Work out the finished part from the listing and answer in its coordinate system (mm). A direction names the side the tool comes from. Round coordinates to 2 decimals unless told otherwise and drop trailing zeros. Order: outer loops, then holes, each group sorted by start corner. A loop starts at its lowest first (then second) coordinate and runs counter-clockwise, first axis right, second up. Notation, with made-up numbers: (-4.75, -14.5) - (36.25, -14.5) arc R32 cw to (36.25, 14.5) - close; hole circle Ø5 at (3, 74). An arc over 180 degrees is marked (long way). Put each result on its own line as item: value.
```python
from build123d import *

# Parameters (mm, degrees)
CROQUIS1_W              = 55
CROQUIS1_H              = 55
SALIENTE_EXTRUIR1_DEPTH = 180
CROQUIS2_R              = 6
CORTAR_EXTRUIR1_DEPTH   = 30
CROQUIS3_R              = 4
CORTAR_EXTRUIR2_DEPTH   = 25
CROQUIS4_R              = 2.5
CORTAR_EXTRUIR3_DEPTH   = 15
CORTAR_EXTRUIR4_START   = -15
CROQUIS5_R              = 2.5
CORTAR_EXTRUIR4_DEPTH   = 15
CROQUIS6_R              = 6
CORTAR_EXTRUIR5_DEPTH   = 12
CHAFL_N1_SIZE           = 2


with BuildPart() as part:
    # Croquis1 → Saliente-Extruir1 (new body)
    with BuildSketch(Plane.XY):
        Rectangle(CROQUIS1_W, CROQUIS1_H)
    extrude(amount=-SALIENTE_EXTRUIR1_DEPTH)

    # Croquis2 → Cortar-Extruir1 (cut)
    with BuildSketch(Plane.XY):
        Circle(CROQUIS2_R)
    extrude(amount=-CORTAR_EXTRUIR1_DEPTH, mode=Mode.SUBTRACT)

    # Croquis3 → Cortar-Extruir2 (cut)
    with BuildSketch(Plane(origin=(0, 0, -180), x_dir=(-1, 0, 0), z_dir=(0, 0, -1))):
        with Locations((18, 18)):
            Circle(CROQUIS3_R)
        with Locations((-18, 18)):
            Circle(CROQUIS3_R)
        with Locations((-18, -18)):
            Circle(CROQUIS3_R)
        with Locations((18, -18)):
            Circle(CROQUIS3_R)
    extrude(amount=-CORTAR_EXTRUIR2_DEPTH, mode=Mode.SUBTRACT)

    # Croquis4 → Cortar-Extruir3 (cut)
    with BuildSketch(Plane(origin=(27.5, 0, 0), x_dir=(0, 0, -1), z_dir=(1, 0, 0))):
        with Locations(Location((18, 21.5, 0), (0, 0, 90))):
            Circle(CROQUIS4_R)
        with Locations(Location((40, 21.5, 0), (0, 0, 90))):
            Circle(CROQUIS4_R)
        with Locations(Location((40, -21.5, 0), (0, 0, 90))):
            Circle(CROQUIS4_R)
        with Locations(Location((18, -21.5, 0), (0, 0, 90))):
            Circle(CROQUIS4_R)
    extrude(amount=-CORTAR_EXTRUIR3_DEPTH, mode=Mode.SUBTRACT)

    # Croquis5 → Cortar-Extruir4 (cut)
    with BuildSketch(Plane.ZY.offset(27.5).offset(CORTAR_EXTRUIR4_START)):
        with Locations(Location((-18, 21.5, 0), (0, 0, 90))):
            Circle(CROQUIS5_R)
        with Locations(Location((-40, 21.5, 0), (0, 0, 90))):
            Circle(CROQUIS5_R)
        with Locations(Location((-40, -21.5, 0), (0, 0, 90))):
            Circle(CROQUIS5_R)
        with Locations(Location((-18, -21.5, 0), (0, 0, 90))):
            Circle(CROQUIS5_R)
    extrude(amount=CORTAR_EXTRUIR4_DEPTH, mode=Mode.SUBTRACT)

    # Croquis6 → Cortar-Extruir5 (cut)
    with BuildSketch(Plane(origin=(0, 27.5, 0), x_dir=(1, 0, 0), z_dir=(0, 1, 0))):
        with Locations(Location((-18, 140, 0), (0, 0, 270))):
            Circle(CROQUIS6_R)
        with Locations(Location((18, 140, 0), (0, 0, 270))):
            Circle(CROQUIS6_R)
    extrude(amount=-CORTAR_EXTRUIR5_DEPTH, mode=Mode.SUBTRACT)

    # Chaflán1
    chafl_n1_edges = [part.edges().sort_by_distance(p)[0] for p in [
        (0, -27.5, 0),
        (-27.5, 0, 0),
        (0, 27.5, 0),
        (27.5, 0, 0),
    ]]
    chamfer(chafl_n1_edges, length=CHAFL_N1_SIZE)


solid = part.part
```
1) A cutting plane is placed at C-C on x = 18. Write down the section's boundary in (y, z).
Findings below:
outline: (-27.5, -180) - (-22, -180) - (-22, -155) - (-14, -155) - (-14, -180) - (14, -180) - (14, -155) - (22, -155) - (22, -180) - (27.5, -180) - (27.5, -146) - (15.5, -146) - (15.5, -134) - (27.5, -134) - (27.5, -2) - (25.5, 0) - (-25.5, 0) - (-27.5, -2) - close; hole circle Ø5 at (-21.5, -40); hole circle Ø5 at (-21.5, -18); hole circle Ø5 at (21.5, -40); hole circle Ø5 at (21.5, -18)
2) A cutting plane is placed at A-A on z = -157. Write down the section's boundary in (x, y).
Findings below:
outline: (-27.5, -27.5) - (27.5, -27.5) - (27.5, 27.5) - (-27.5, 27.5) - close; hole circle Ø8 at (-18, -18); hole circle Ø8 at (-18, 18); hole circle Ø8 at (18, -18); hole circle Ø8 at (18, 18)
3) Straight lines are drawn through the part: L1, parallel to Y at x = -15, z = -40; L2, parallel to Y at x = -18, z = -166; L3, parallel to X at y = -15.5, z = -158.5. For each, find the intervals that lie inside material, in ascending order. Write a range as from..to.
Findings below:
L1: y = -27.5..-24, -19..19, 24..27.5
L2: y = -27.5..-22, -14..14, 22..27.5
L3: x = -27.5..-21.12, -14.88..14.88, 21.12..27.5
4) A cutting plane is placed at B-B on y = 0. Write down the section's boundary in (x, z).
Findings below:
outline: (-27.5, -180) - (27.5, -180) - (27.5, -2) - (25.5, 0) - (6, 0) - (6, -30) - (-6, -30) - (-6, 0) - (-25.5, 0) - (-27.5, -2) - close
5) Given pin 1 Ø6 at (y, z) = (21.5, -40) entering from -X; pin 2 Ø1.5 at (y, z) = (21, -40.5) entering from +X; pin 3 Ø3.5 at (x, z) = (-18.5, -140.5) entering from +Y; pin 4 Ø4.5 at (y, z) = (21.5, -18) entering from -X, each flat-ended and moving along its own axis, determine where each tip first touches the part or whether it passes through.
Findings below:
pin 1: stops at x = -27.5
pin 2: stops at x = 12.5
pin 3: stops at y = 15.5
pin 4: stops at x = -12.5
6) For faces 1 (the flat face through (12.5, 21, -40)), 2 (the cylindrical face through (-20, 20, -38)), 3 (the flat face through (0, 0, -30)), 4 (the cylindrical face through (14.35, 21.58, -144.76)), 5 (the flat face through (-18, 18, -155)), determine the directions among +Z, -Z, +X, -X, +Y, -Y from which every point of the face is accessible in a straight line to the end or side of a thin tool.
Findings below:
face 1: +X
face 2: -X
face 3: +Z
face 4: +Y
face 5: -Z
7) A cutting plane is placed at D-D on z = -27. Write down the section's boundary in (x, y).
Findings below:
outline: (-27.5, -27.5) - (27.5, -27.5) - (27.5, 27.5) - (-27.5, 27.5) - close; hole circle Ø12 at (0, 0)
8) For a pull along Y with two mould halves and no side action, classify faces 6 (the flat face through (18, -18, -155)), 7 (the cylindrical face through (-20, 20, -20)), 8 (the flat face through (27.5, 0, -90)) as pulls with the +Y half, pulls with the -Y half, needs draft (parallel to the pull), parting line crosses it, or undercut.
Findings below:
face 6: undercut
face 7: undercut
face 8: needs draft
